```python
from build123d import *

# Parameters (mm, degrees)
F2_SIZE  = 1
F3_SIZE  = 2
F5_DEPTH = 100


with BuildPart() as f1:
    # F0 (on Front) → F1 (revolve)
    with BuildSketch(Plane.XZ):
        Polygon((237.5, -103.5), (237.5, 0), (228, 0), (228, -8), (230, -8), (230, -18), (228, -18), (228, -25.5), (218, -25.5), (218, -40.5), (224, -40.5), (224, -78.5), (233, -78.5), (233, -98.5), (224, -98.5), (224, -103.5), align=None)
    revolve(axis=Axis((0, 0, -40.326346), (0, 0, -1)))

    # F2
    f2_edges = [f1.edges().sort_by_distance(p)[0] for p in [
        (-228, 0, 0),
    ]]
    chamfer(f2_edges, length=F2_SIZE)

    # F3
    f3_edges = [f1.edges().sort_by_distance(p)[0] for p in [
        (-237.5, 0, 0),
        (-224, 0, -103.5),
        (-237.5, 0, -103.5),
    ]]
    chamfer(f3_edges, length=F3_SIZE)

    # F4 (on Top) → F5 (cut, symmetric)
    with BuildSketch(Plane.XY):
        with BuildLine():
            ThreePointArc((-24.999351, 216.561844), (0, 218), (24.999351, 216.561844))
            ThreePointArc((24.999351, 216.561844), (0, 224), (-24.999351, 216.561844))
        make_face()
        with BuildLine():
            ThreePointArc((-24.999351, -216.561844), (0, -224), (24.999351, -216.561844))
            ThreePointArc((24.999351, -216.561844), (0, -218), (-24.999351, -216.561844))
        make_face()
    extrude(amount=F5_DEPTH, both=True, mode=Mode.SUBTRACT)


solid = f1.part
```
Input: part model. Units: mm. Frame: model coordinates. A direction names the side the tool comes from. Give positions to 0.01 mm unless a question says otherwise; leave off trailing zeros. Order: outer loops, then holes, each group sorted by start corner. A loop starts at its lowest first (then second) coordinate and runs counter-clockwise, first axis right, second up. Notation, with made-up numbers: M 55.25,81.25 L 99.25,81.25 A24 ccw 99.25,96.25 Z; hole C -39.5,17.5 d7. An arc over 180 degrees is marked long. Return JSON: item names as keys, results as strings.
1) Line query: L1, parallel to Y at x = 0, z = -85; L2, parallel to X at y = 0, z = -23.5. Output: solid intervals per line, ascending. Write a range as [from, to].
Taken from the geometry:
{"L1": "y = [-237.5, -233], [233, 237.5]", "L2": "x = [-237.5, -228], [228, 237.5]"}
2) Mould query, pull axis X, two halves, no side actions, for faces 6 (the face through (51, 226, 0)), 7 (the face through (-51.079, 230.022, -0.125)), 8 (the face through (52, -223, -8)). Classes: released by +X, released by -X, zero draft, split by the parting line, or undercut.
Taken from the geometry:
{"face 6": "zero draft", "face 7": "split by the parting line", "face 8": "undercut"}
3) Contact query for flat-ended pins moving along their axis: pin 1 (12 mm diameter, centred on y = 112.5, z = -55.5, fed in from -X); pin 2 (1 mm diameter, centred on y = 88.5, z = -14.5, fed in from +X); pin 3 (6 mm diameter, centred on y = -93, z = -88.5, fed in from +X). Output: stop coordinate, or through.
Taken from the geometry:
{"pin 1": "stops at x = -212.28", "pin 2": "stops at x = 220.6", "pin 3": "stops at x = 219.79"}
4) Access query for faces 1 (the face through (210.61, 87.33, -21.8)), 2 (the face through (210, -88, -103.5)), 3 (the face through (206.92, 85.79, -100.02)), 4 (the face through (-49.86, 224.53, -13.07)), 5 (the face through (0, 224, -33)). Directions: +Z, -Z, +X, -X, +Y, -Y. A direction counts if a zero-diameter tool reaches every point of the face in a straight line with its end or side. Return the directions, or none.
Taken from the geometry:
{"face 1": "+Z", "face 2": "-Z, +X, -X, +Y, -Y", "face 3": "-Z", "face 4": "none", "face 5": "+Z, -Z"}
5) Section query A-A on z = -69.5. Output: boundary loops of the cut face in (x, y).
Taken from the geometry:
{"outline": "C 0,0 d475; hole C 0,0 d448"}
